Could you check a few things on this model? Use its own coordinates, in mm. A direction names the side the tool comes from. Give positions to 0.01 mm unless a question says otherwise; leave off trailing zeros. One line per question, with ' | ' between items. Start each with the question number.
1. For P1, Ø2, axis at y = 6, z = -9.5, coming from the -X side; P2, Ø1, axis at x = -4.5, y = 7.5, coming from the -Z side; P3, Ø1.6, axis at y = 9.19, z = -11.82, coming from the -X side, each with a flat end and sliding along its axis, tell me the tip position at first contact or that it passes through.
2. I need wall thicknesses on probe 1 along X at (y, z) = (11.5, 9); probe 2 along X at (y, z) = (8.75, -11); probe 3 along Z at (x, y) = (11, 11.75). Which ranges of each line are inside material? Lowest first, please. Write a range as from..to.
3. Which directions (+Z, -Z, +X, -X, +Y, -Y) give clear straight access to the entire face, cutting with the end or side of a thin tool? Please do faces 4 (the flat face through (-3.947, 10.459, -5.069)), 5 (the flat face through (8.64, 5.79, -4.91)), 6 (the flat face through (3.526, 10.902, -5.649)).
4. If we mould it in two halves opening along X, with no side actions, what happens to faces 1 (the flat face through (-4.536, 2.336, -2.817)), 2 (the flat face through (-7.55, 7.09, -9.7)), 3 (the flat face through (12.455, 8.618, 3.896))? For each: released by +X, released by -X, zero draft, split by the parting line, or undercut.
```python
from build123d import *

# Parameters (mm, degrees)
BOSS_EXTRUDE1_DEPTH     = 6.752040791
BOSS_EXTRUDE1_TAPER     = 31.717474411
SKETCH3_R               = 1
CUT_EXTRUDE1_DEPTH      = 2
CIRPATTERN1_COUNT       = 5
MIRROR3_COPY_1_SKETCH_R = 1
MIRROR3_COPY_1_DEPTH    = 2
MIRROR3_COPY_2_SKETCH_R = 1
MIRROR3_COPY_2_DEPTH    = 2
MIRROR3_COPY_3_SKETCH_R = 1
MIRROR3_COPY_3_DEPTH    = 2
MIRROR3_COPY_4_SKETCH_R = 1
MIRROR3_COPY_4_DEPTH    = 2
MIRROR4_COPY_1_SKETCH_R = 1
MIRROR4_COPY_1_DEPTH    = 2
MIRROR4_COPY_2_SKETCH_R = 1
MIRROR4_COPY_2_DEPTH    = 2
MIRROR4_COPY_3_SKETCH_R = 1
MIRROR4_COPY_3_DEPTH    = 2
MIRROR4_COPY_4_SKETCH_R = 1
MIRROR4_COPY_4_DEPTH    = 2
MIRROR5_COPY_1_SKETCH_R = 1
MIRROR5_COPY_1_DEPTH    = 2
MIRROR5_COPY_2_SKETCH_R = 1
MIRROR5_COPY_2_DEPTH    = 2
MIRROR5_COPY_3_SKETCH_R = 1
MIRROR5_COPY_3_DEPTH    = 2
MIRROR5_COPY_4_SKETCH_R = 1
MIRROR5_COPY_4_DEPTH    = 2


with BuildPart() as part:
    # Sketch1 → Boss-Extrude1 (new body)
    with BuildSketch(Plane(origin=(0, 0, 0), x_dir=(1, 0, 0), z_dir=(0, 1, 0))):
        Polygon((0, 10.803265266), (-10.274515829, 3.338392562), (-6.35, -8.740025195), (6.35, -8.740025195), (10.274515829, 3.338392562), align=None)
    boss_extrude1 = extrude(amount=BOSS_EXTRUDE1_DEPTH, taper=BOSS_EXTRUDE1_TAPER)

    # Sketch3 → Cut-Extrude1 (cut)
    with BuildSketch(Plane(origin=(0, 3.908658092, 6.324341644), x_dir=(1, 0, 0), z_dir=(1.6266940928737823e-15, 0.5257311121191348, 0.8506508083520392))):
        with Locations(Location((-2, -0.626153166, 0), (0, 0, 270))):
            Circle(SKETCH3_R)
        with Locations(Location((2, -0.626153166, 0), (0, 0, 270))):
            Circle(SKETCH3_R)
    cut_extrude1 = extrude(amount=-CUT_EXTRUDE1_DEPTH, mode=Mode.SUBTRACT)

    # CirPattern1: Cut-Extrude1 ×5 about axis
    cirpattern1_axis = Axis((0, 0, 0), (0, 1, 0))
    for i in range(1, CIRPATTERN1_COUNT):
        add(cut_extrude1.rotate(cirpattern1_axis, i * 360 / CIRPATTERN1_COUNT), mode=Mode.SUBTRACT)

    # Mirror3: Boss-Extrude1, Cut-Extrude1 across plane
    add(boss_extrude1.mirror(Plane(origin=(10.274515829, 0, -3.338392562), x_dir=(0.4742680099309791, 0.49867489660708614, 0.7255296012224591), z_dir=(0.4999999999999987, 0.5257311121191346, -0.688190960235587))))
    add(cut_extrude1.mirror(Plane(origin=(10.274515829, 0, -3.338392562), x_dir=(0.4742680099309791, 0.49867489660708614, 0.7255296012224591), z_dir=(0.4999999999999987, 0.5257311121191346, -0.688190960235587))), mode=Mode.SUBTRACT)

    # Mirror3 copy 1 sketch → Mirror3 copy 1 (cut)
    with BuildSketch(Plane(origin=(9.73216108, 7.817316184, -3.162170822), x_dir=(-0.49999999999999817, -0.8506508083520414, 0.16245984811645184), z_dir=(0.3090169943749473, -1.0229261620413978e-15, 0.9510565162951535))):
        with Locations((-2, 0.626153166)):
            Circle(MIRROR3_COPY_1_SKETCH_R)
        with Locations((2, 0.626153166)):
            Circle(MIRROR3_COPY_1_SKETCH_R)
    extrude(amount=-MIRROR3_COPY_1_DEPTH, mode=Mode.SUBTRACT)

    # Mirror3 copy 2 sketch → Mirror3 copy 2 (cut)
    with BuildSketch(Plane(origin=(3.717354749, 3.908658092, -5.116499868), x_dir=(-0.8090169943749478, 0, -0.5877852522924726), z_dir=(-0.49999999999999917, -0.5257311121191345, 0.688190960235587))):
        with Locations((-2, 0.626153166)):
            Circle(MIRROR3_COPY_2_SKETCH_R)
        with Locations((2, 0.626153166)):
            Circle(MIRROR3_COPY_2_SKETCH_R)
    extrude(amount=-MIRROR3_COPY_2_DEPTH, mode=Mode.SUBTRACT)

    # Mirror3 copy 3 sketch → Mirror3 copy 3 (cut)
    with BuildSketch(Plane(origin=(0, 7.817316184, -10.232999736), x_dir=(-1.481930376076656e-15, 0.8506508083520405, -0.5257311121191328), z_dir=(-1, 0, 0))):
        with Locations((-2, 0.626153166)):
            Circle(MIRROR3_COPY_3_SKETCH_R)
        with Locations((2, 0.626153166)):
            Circle(MIRROR3_COPY_3_SKETCH_R)
    extrude(amount=-MIRROR3_COPY_3_DEPTH, mode=Mode.SUBTRACT)

    # Mirror3 copy 4 sketch → Mirror3 copy 4 (cut)
    with BuildSketch(Plane(origin=(3.717354749, 14.141657828, -11.440841512), x_dir=(0.8090169943749475, 0.525731112119134, 0.2628655560595658), z_dir=(-0.5000000000000016, 0.8506508083520398, -0.16245984811644956))):
        with Locations((-2, 0.626153166)):
            Circle(MIRROR3_COPY_4_SKETCH_R)
        with Locations((2, 0.626153166)):
            Circle(MIRROR3_COPY_4_SKETCH_R)
    extrude(amount=-MIRROR3_COPY_4_DEPTH, mode=Mode.SUBTRACT)

    # Mirror4: Boss-Extrude1, Cut-Extrude1 across plane
    add(boss_extrude1.mirror(Plane(origin=(6.35, 0, 8.740025195), x_dir=(-0.22041412184245382, -0.1432337790289861, 0.9648324722134385), z_dir=(0.8090169943749472, 0.5257311121191346, 0.26286555605956535))))
    add(cut_extrude1.mirror(Plane(origin=(6.35, 0, 8.740025195), x_dir=(-0.22041412184245382, -0.1432337790289861, 0.9648324722134385), z_dir=(0.8090169943749472, 0.5257311121191346, 0.26286555605956535))), mode=Mode.SUBTRACT)

    # Mirror4 copy 1 sketch → Mirror4 copy 1 (cut)
    with BuildSketch(Plane(origin=(6.014806331, 3.908658092, 1.954329046), x_dir=(0.30901699437494656, 0, -0.9510565162951539), z_dir=(-0.8090169943749472, -0.5257311121191344, -0.26286555605956563))):
        with Locations((-2, 0.626153166)):
            Circle(MIRROR4_COPY_1_SKETCH_R)
        with Locations((2, 0.626153166)):
            Circle(MIRROR4_COPY_1_SKETCH_R)
    extrude(amount=-MIRROR4_COPY_1_DEPTH, mode=Mode.SUBTRACT)

    # Mirror4 copy 2 sketch → Mirror4 copy 2 (cut)
    with BuildSketch(Plane(origin=(9.73216108, 7.817316184, -3.162170822), x_dir=(0.49999999999999856, 0.8506508083520403, -0.16245984811645464), z_dir=(-0.30901699437494995, 0, -0.9510565162951526))):
        with Locations((-2, 0.626153166)):
            Circle(MIRROR4_COPY_2_SKETCH_R)
        with Locations((2, 0.626153166)):
            Circle(MIRROR4_COPY_2_SKETCH_R)
    extrude(amount=-MIRROR4_COPY_2_DEPTH, mode=Mode.SUBTRACT)

    # Mirror4 copy 3 sketch → Mirror4 copy 3 (cut)
    with BuildSketch(Plane(origin=(12.029612663, 14.141657828, 0), x_dir=(1.0269562977782761e-15, 0.5257311121191341, 0.8506508083520397), z_dir=(-4.107825191113078e-15, 0.8506508083520397, -0.5257311121191341))):
        with Locations((-2, 0.626153166)):
            Circle(MIRROR4_COPY_3_SKETCH_R)
        with Locations((2, 0.626153166)):
            Circle(MIRROR4_COPY_3_SKETCH_R)
    extrude(amount=-MIRROR4_COPY_3_DEPTH, mode=Mode.SUBTRACT)

    # Mirror4 copy 4 sketch → Mirror4 copy 4 (cut)
    with BuildSketch(Plane(origin=(9.73216108, 14.141657828, 7.070828914), x_dir=(-0.49999999999999695, -0.5257311121191343, 0.6881909602355885), z_dir=(-0.30901699437494995, 0.8506508083520394, 0.4253254041760191))):
        with Locations((-2, 0.626153166)):
            Circle(MIRROR4_COPY_4_SKETCH_R)
        with Locations((2, 0.626153166)):
            Circle(MIRROR4_COPY_4_SKETCH_R)
    extrude(amount=-MIRROR4_COPY_4_DEPTH, mode=Mode.SUBTRACT)

    # Mirror5: Boss-Extrude1, Cut-Extrude1 across plane
    add(boss_extrude1.mirror(Plane(origin=(0, 0, -10.803265266), x_dir=(-0.4742680099309791, 0.49867489660708403, 0.7255296012224607), z_dir=(-0.5000000000000008, 0.5257311121191346, -0.6881909602355855))))
    add(cut_extrude1.mirror(Plane(origin=(0, 0, -10.803265266), x_dir=(-0.4742680099309791, 0.49867489660708403, 0.7255296012224607), z_dir=(-0.5000000000000008, 0.5257311121191346, -0.6881909602355855))), mode=Mode.SUBTRACT)

    # Mirror5 copy 1 sketch → Mirror5 copy 1 (cut)
    with BuildSketch(Plane(origin=(-3.717354749, 14.141657828, -11.440841512), x_dir=(0.809016994374946, -0.5257311121191343, -0.2628655560595699), z_dir=(0.5000000000000014, 0.8506508083520394, -0.16245984811645112))):
        with Locations((-2, 0.626153166)):
            Circle(MIRROR5_COPY_1_SKETCH_R)
        with Locations((2, 0.626153166)):
            Circle(MIRROR5_COPY_1_SKETCH_R)
    extrude(amount=-MIRROR5_COPY_1_DEPTH, mode=Mode.SUBTRACT)

    # Mirror5 copy 2 sketch → Mirror5 copy 2 (cut)
    with BuildSketch(Plane(origin=(0, 7.817316184, -10.232999736), x_dir=(0, -0.8506508083520414, 0.5257311121191313), z_dir=(1, 0, 0))):
        with Locations((-2, 0.626153166)):
            Circle(MIRROR5_COPY_2_SKETCH_R)
        with Locations((2, 0.626153166)):
            Circle(MIRROR5_COPY_2_SKETCH_R)
    extrude(amount=-MIRROR5_COPY_2_DEPTH, mode=Mode.SUBTRACT)

    # Mirror5 copy 3 sketch → Mirror5 copy 3 (cut)
    with BuildSketch(Plane(origin=(-3.717354749, 3.908658092, -5.116499868), x_dir=(-0.8090169943749468, 0, 0.5877852522924741), z_dir=(0.5000000000000007, -0.5257311121191344, 0.6881909602355856))):
        with Locations((-2, 0.626153166)):
            Circle(MIRROR5_COPY_3_SKETCH_R)
        with Locations((2, 0.626153166)):
            Circle(MIRROR5_COPY_3_SKETCH_R)
    extrude(amount=-MIRROR5_COPY_3_DEPTH, mode=Mode.SUBTRACT)

    # Mirror5 copy 4 sketch → Mirror5 copy 4 (cut)
    with BuildSketch(Plane(origin=(-9.73216108, 7.817316184, -3.162170822), x_dir=(-0.49999999999999994, 0.8506508083520404, -0.16245984811645106), z_dir=(-0.30901699437494473, 0, 0.9510565162951545))):
        with Locations((-2, 0.626153166)):
            Circle(MIRROR5_COPY_4_SKETCH_R)
        with Locations((2, 0.626153166)):
            Circle(MIRROR5_COPY_4_SKETCH_R)
    extrude(amount=-MIRROR5_COPY_4_DEPTH, mode=Mode.SUBTRACT)


solid = part.part
```
Results found:
1) P1: stops at x = -8.52 | P2: stops at z = -12.65 | P3: stops at x = -7.71
2) probe 1: x = 6.54..9.17, 10.18..12.31 | probe 2: x = -7.17..-2, 2..7.17 | probe 3: z = -10.07..-7.77, -5.62..12.78
3) face 4: +Z, +Y | face 5: none | face 6: +Y
4) face 1: undercut | face 2: released by -X | face 3: released by +X
